Check sheet for the modelled part. Datum: model origin and axes. Units: mm. Give positions to 0.01 mm unless a question says otherwise; leave off trailing zeros. Write each loop counter-clockwise with the first axis right and the second up, starting at its lowest first coordinate (ties: lowest second). Pieces come first, ordered by that corner, then holes. Notation, with made-up numbers: (-5, -19) -> (32, -19) arc R23 cw to (32, 14) -> close; hole circle Ø3 at (37.25, 41). An arc over 180 degrees is marked (long way). Use a Markdown table: item, result. Add a question column.
1. Cross-section at D-D (x = 1.95). Enter the section's corners in (y, z), then the cut area to 3 significant figures.
2. Cross-section at C-C (y = -2.5). Enter the section's corners in (x, z), then the cut area to 3 significant figures.
3. Cross-section at B-B (y = -1.75). Enter the section's corners in (x, z), then the cut area to 3 significant figures.
4. Scan lines: probe 1 along X at (y, z) = (0.05, 8.75); probe 2 along Z at (x, y) = (-1.8, -1.15); probe 3 along Y at (x, z) = (2.05, 6). Record each from-to range of solid material in increasing order. Write a range as [from, to].
5. Gauge pin test, flat ends, axial feed: P1, Ø1, axis at x = 0.5, y = -2, coming from the -Z side; P2, Ø1.5, axis at y = 0, z = 4, coming from the -X side. Record the tip position at first contact, or that the pin passes through.
6. Release check for a two-part mould opening along Y. For faces 1 (the flat face through (0, 2.9, 1)), 2 (the flat face through (0, -2.1, 5)), 3 (the flat face through (0, -2.1, 10)), 4 (the flat face through (2.54, -1, 2)) record: released by +Y, released by -Y, zero draft, split by the parting line, or undercut.
7. Cross-section at A-A (z = 9.5). Enter the section's corners in (x, y).
from build123d import *

# Parameters (mm, degrees)
SKETCH_1_W             = 5.08
SKETCH_1_H             = 5.8
EXTRUDE_1_DEPTH        = 11.7
CUT_EXTRUDE_1_DEPTH    = 14.080764504
EXTRUDE_START          = -10
EXTRUDE_2_DEPTH        = 12
FILLET_1_R             = 0.1
FILLET_2_R             = 0.1
FILLET_1_OF_MIRROR_2_R = 0.1


with BuildPart() as part:
    # 草图1 → 凸台-拉伸1 (new body)
    with BuildSketch(Plane.XY):
        Rectangle(SKETCH_1_W, SKETCH_1_H)
    extrude(amount=EXTRUDE_1_DEPTH)

    # 草图2 → 切除-拉伸1 (cut, through all)
    with BuildSketch(Plane(origin=(2.54, 0, 0), x_dir=(0, 0, -1), z_dir=(1, 0, 0))):
        Polygon((-11.7, -2.1), (-8, -2.1), (-7.5, -1.6), (-7, -1.6), (-7, -2.1), (-3, -2.1), (-3, 2.9), (-11.7, 2.9), align=None)
    extrude(amount=-CUT_EXTRUDE_1_DEPTH, mode=Mode.SUBTRACT)

    # 草图3 → 凸台-拉伸2 (add)
    with BuildSketch(Plane(origin=(0, 0, 0), x_dir=(-1, 0, 0), z_dir=(0, 0, -1)).offset(EXTRUDE_START)):
        with BuildLine():
            Line((-1.57, -0.15), (-1.57, 0.15))
            ThreePointArc((-1.57, 0.15), (-1.526066017, 0.256066017), (-1.42, 0.3))
            Line((-1.42, 0.3), (-1.12, 0.3))
            ThreePointArc((-1.12, 0.3), (-1.013933983, 0.256066017), (-0.97, 0.15))
            Line((-0.97, 0.15), (-0.97, -0.15))
            ThreePointArc((-0.97, -0.15), (-1.013933983, -0.256066017), (-1.12, -0.3))
            Line((-1.12, -0.3), (-1.42, -0.3))
            ThreePointArc((-1.42, -0.3), (-1.526066017, -0.256066017), (-1.57, -0.15))
        make_face()
    extrude_2 = extrude(amount=EXTRUDE_2_DEPTH)

    # 圆角1
    fillet_1_edges = [part.edges().sort_by_distance(p)[0] for p in [
        (1.013933983, 0.256066017, 10),
        (0.97, 0, 10),
        (1.013933983, -0.256066017, 10),
        (1.27, -0.3, 10),
        (1.526066017, -0.256066017, 10),
        (1.57, 0, 10),
        (1.526066017, 0.256066017, 10),
        (1.27, 0.3, 10),
        (1.013933983, 0.256066017, -2),
        (1.27, 0.3, -2),
        (1.526066017, 0.256066017, -2),
        (1.57, 0, -2),
        (1.526066017, -0.256066017, -2),
        (1.27, -0.3, -2),
        (1.013933983, -0.256066017, -2),
        (0.97, 0, -2),
    ]]
    fillet(fillet_1_edges, radius=FILLET_1_R)

    # 圆角2
    fillet_2_edges = [part.edges().sort_by_distance(p)[0] for p in [
        (0, -2.9, 11.7),
        (-2.54, -2.5, 11.7),
        (-2.54, 2.9, 1.5),
        (2.54, 2.9, 1.5),
        (0, -2.1, 11.7),
        (-2.54, 0.4, 3),
        (0, 2.9, 3),
        (-2.54, -2.1, 5),
        (0, -2.1, 3),
        (-2.54, -2.1, 9.85),
        (2.54, -2.1, 9.85),
        (2.54, -2.1, 5),
        (2.54, 0.4, 3),
        (2.54, -2.5, 11.7),
        (0, -2.9, 0),
        (-2.54, 0, 0),
        (0, 2.9, 0),
        (2.54, 0, 0),
        (2.54, -2.9, 5.85),
        (-2.54, -2.9, 5.85),
    ]]
    fillet(fillet_2_edges, radius=FILLET_2_R)

    # 镜向2: 凸台-拉伸2 across plane
    add(extrude_2.mirror(Plane(origin=(0, 0, 0), x_dir=(0, 0, 1), z_dir=(1, 0, 0))))

    # 圆角1 of 镜向2
    fillet_1_of_mirror_2_edges = [part.edges().sort_by_distance(p)[0] for p in [
        (-1.013933983, 0.256066017, 10),
        (-0.97, 0, 10),
        (-1.013933983, -0.256066017, 10),
        (-1.27, -0.3, 10),
        (-1.526066017, -0.256066017, 10),
        (-1.57, 0, 10),
        (-1.526066017, 0.256066017, 10),
        (-1.27, 0.3, 10),
        (-1.013933983, 0.256066017, -2),
        (-1.27, 0.3, -2),
        (-1.526066017, 0.256066017, -2),
        (-1.57, 0, -2),
        (-1.526066017, -0.256066017, -2),
        (-1.27, -0.3, -2),
        (-1.013933983, -0.256066017, -2),
        (-0.97, 0, -2),
    ]]
    fillet(fillet_1_of_mirror_2_edges, radius=FILLET_1_OF_MIRROR_2_R)


solid = part.part
Worked answers:
| question | item | result |
|---|---|---|
| 1 | outline | (-2.9, 0.1) arc R0.1 ccw to (-2.8, 0) -> (2.8, 0) arc R0.1 ccw to (2.9, 0.1) -> (2.9, 2.9) arc R0.1 ccw to (2.8, 3) -> (-2, 3) arc R0.1 cw to (-2.1, 3.1) -> (-2.1, 7) -> (-1.6, 7) -> (-1.6, 7.5) -> (-2.1, 8) -> (-2.1, 11.6) arc R0.1 ccw to (-2.2, 11.7) -> (-2.8, 11.7) arc R0.1 ccw to (-2.9, 11.6) -> close |
| 1 | area | 24.7 mm² |
| 2 | outline | (-2.54, 0.1) arc R0.1 ccw to (-2.44, 0) -> (2.44, 0) arc R0.1 ccw to (2.54, 0.1) -> (2.54, 11.6) arc R0.1 ccw to (2.44, 11.7) -> (-2.44, 11.7) arc R0.1 ccw to (-2.54, 11.6) -> close |
| 2 | area | 59.4 mm² |
| 3 | outline | (-2.54, 0.1) arc R0.1 ccw to (-2.44, 0) -> (2.44, 0) arc R0.1 ccw to (2.54, 0.1) -> (2.54, 2.9) arc R0.1 ccw to (2.44, 3) -> (-2.44, 3) arc R0.1 ccw to (-2.54, 2.9) -> close; (-2.54, 7) -> (2.54, 7) -> (2.54, 7.65) -> (-2.54, 7.65) -> close |
| 3 | area | 18.5 mm² |
| 4 | probe 1 | x = [-1.57, -0.97], [0.97, 1.57] |
| 4 | probe 2 | z = [0, 3] |
| 4 | probe 3 | y = [-2.9, -2.1] |
| 5 | P1 | stops at z = 0 |
| 5 | P2 | stops at x = -1.57 |
| 6 | face 1 | released by +Y |
| 6 | face 2 | undercut |
| 6 | face 3 | undercut |
| 6 | face 4 | zero draft |
| 7 | outline | (-2.54, -2.8) arc R0.1 ccw to (-2.44, -2.9) -> (2.44, -2.9) arc R0.1 ccw to (2.54, -2.8) -> (2.54, -2.2) arc R0.1 ccw to (2.44, -2.1) -> (-2.44, -2.1) arc R0.1 ccw to (-2.54, -2.2) -> close; (-1.57, -0.15) arc R0.15 ccw to (-1.42, -0.3) -> (-1.12, -0.3) arc R0.15 ccw to (-0.97, -0.15) -> (-0.97, 0.15) arc R0.15 ccw to (-1.12, 0.3) -> (-1.42, 0.3) arc R0.15 ccw to (-1.57, 0.15) -> close; (0.97, -0.15) arc R0.15 ccw to (1.12, -0.3) -> (1.42, -0.3) arc R0.15 ccw to (1.57, -0.15) -> (1.57, 0.15) arc R0.15 ccw to (1.42, 0.3) -> (1.12, 0.3) arc R0.15 ccw to (0.97, 0.15) -> close |
